Work out the finished part from the listing and answer in its coordinate system (mm). A direction names the side the tool comes from. Coordinates: 2 decimals unless noted, no trailing zeros. Order: outer loops, then holes, each group sorted by start corner. A loop starts at its lowest first (then second) coordinate and runs counter-clockwise, first axis right, second up.
1. Flat-ended cylindrical pins translate along their axes: pin 1 Ø1 at (x, y) = (26, -37) entering from -Z; pin 2 Ø6 at (x, z) = (-18.5, 24.5) entering from +Y; pin 3 Ø1.9 at (y, z) = (-31, 22) entering from -X; pin 4 Ø12 at (x, z) = (22.5, 22) entering from +Y. Find the tip coordinate at first contact, or state that the pin passes through.
2. The part is cut by section B-B, the plane z = 12.5. Give the vertices of the cut face in (x, y).
3. Find the intervals of material crossed by probe 1 along X at (y, z) = (-38, 7); probe 2 along X at (y, z) = (-35.75, 7.5); probe 3 along X at (y, z) = (-31, 19.5), in increasing order.
4. Determine the mould class of faces 4 (the flat face through (11, -30, 23)), 5 (the flat face through (0.6, -36.49, 12.92)), 6 (the cylindrical face through (-21.9, -32.5, 19.5)) for opening direction Z: +Z half, -Z half, draft (parallel to the pull), parting line (faces both ways), or undercut.
5. The part is cut by section A-A, the plane x = 3. Give the vertices of the cut face in (y, z), then the cut area to 3 significant figures.
6. A tool of negligible diameter and unlimited length cuts with its end or side. For faces 1 (the conical face through (-13.377, -33.758, 16.894)), 2 (the cylindrical face through (10.323, -32.344, 16.981)), 3 (the conical face through (-13.424, -29.345, 29.017)), from which of +Z, -Z, +X, -X, +Y, -Y can it reach the whole face along a straight path? Write none if from no direction.
```python
from build123d import *

# Parameters (mm, degrees)
SKETCH033_R             = 1.65
SKETCH033_R_2           = 3.7
PAD001_DEPTH            = 3
CHAMFER001_SIZE         = 2
CHAMFER002_SIZE         = 1.4
SKETCH035_R             = 1.5
POCKET009_DEPTH         = 1.5
BODY005_PLACEMENT_ANGLE = 340


with BuildPart() as part:
    # Sketch033 → Pad001 (new body)
    with BuildSketch(Plane.XZ):
        with BuildLine():
            Line((-33.808366, 37.4), (33.808366, 37.4))
            ThreePointArc((41.8, 29.765194), (39.33458, 35.18452), (33.808366, 37.4))
            Line((41.8, 29.765194), (42.65, 11.165194))
            ThreePointArc((34.658366, 2.8), (40.442878, 5.273779), (42.65, 11.165194))
            Line((34.658366, 2.8), (-34.658366, 2.8))
            ThreePointArc((-42.65, 11.165194), (-40.442878, 5.273779), (-34.658366, 2.8))
            Line((-42.65, 11.165194), (-41.8, 29.765194))
            ThreePointArc((-33.808366, 37.4), (-39.33458, 35.18452), (-41.8, 29.765194))
        make_face()
        with Locations((-36.75, 32.1)):
            Circle(SKETCH033_R, mode=Mode.SUBTRACT)
        with Locations((36.75, 32.1)):
            Circle(SKETCH033_R, mode=Mode.SUBTRACT)
        with Locations((-38, 8.1)):
            Circle(SKETCH033_R, mode=Mode.SUBTRACT)
        with Locations((38, 8.1)):
            Circle(SKETCH033_R, mode=Mode.SUBTRACT)
        with Locations((25.5, 23.3)):
            Circle(SKETCH033_R_2, mode=Mode.SUBTRACT)
        with BuildLine():
            Line((-11.25, 30.35), (8.75, 30.35))
            ThreePointArc((11, 28.1), (10.34099, 29.69099), (8.75, 30.35))
            Line((11, 28.1), (11, 19.5))
            ThreePointArc((8.75, 17.25), (10.34099, 17.90901), (11, 19.5))
            Line((8.75, 17.25), (-11.25, 17.25))
            ThreePointArc((-13.5, 19.5), (-12.84099, 17.90901), (-11.25, 17.25))
            Line((-13.5, 19.5), (-13.5, 28.1))
            ThreePointArc((-11.25, 30.35), (-12.84099, 29.69099), (-13.5, 28.1))
        make_face(mode=Mode.SUBTRACT)
        with BuildLine():
            Line((-30.35, 25.929165), (-25.65, 25.929165))
            ThreePointArc((-25.65, 14.670835), (-21.9, 20.3), (-25.65, 25.929165))
            Line((-30.35, 14.670835), (-25.65, 14.670835))
            ThreePointArc((-30.35, 25.929165), (-34.1, 20.3), (-30.35, 14.670835))
        make_face(mode=Mode.SUBTRACT)
    extrude(amount=PAD001_DEPTH)

    # Chamfer001
    chamfer001_edges = [part.edges().sort_by_distance(p)[0] for p in [
        (-1.25, -3, 30.35),
    ]]
    chamfer(chamfer001_edges, length=CHAMFER001_SIZE)

    # Chamfer002
    chamfer002_edges = [part.edges().sort_by_distance(p)[0] for p in [
        (-38.4, -3, 32.1),
        (-39.65, -3, 8.1),
        (35.1, -3, 32.1),
        (36.35, -3, 8.1),
    ]]
    chamfer(chamfer002_edges, length=CHAMFER002_SIZE)

    # Sketch035 → Pocket009 (cut)
    with BuildSketch(Plane.XZ):
        with Locations((25.5, 30.3)):
            Circle(SKETCH035_R)
    extrude(amount=POCKET009_DEPTH, mode=Mode.SUBTRACT)


with BuildPart() as part_1:
    # Body005 placement: moved
    add(part.part.moved(Location((0, -38, 0))).rotate(Axis((0, -38, 0), (1, 0, 0)), BODY005_PLACEMENT_ANGLE))


solid = part_1.part
```
Geometry says:
1. pin 1: stops at z = 2.63
1. pin 2: stops at y = -27.99
1. pin 3: stops at x = -42.15
1. pin 4: stops at y = -27.81
2. outline: (-42.6, -36.64) - (42.6, -36.64) - (42.55, -33.45) - (-42.55, -33.45) - close
3. probe 1: x = -41.45 to -39.91, -36.09 to 36.09, 39.91 to 41.45
3. probe 2: x = -42.08 to -39.63, -36.37 to 36.37, 39.63 to 42.08
3. probe 3: x = -42.21 to -34.09, -21.91 to -13.5, 11 to 22.85, 28.15 to 42.21
4. face 4: draft
4. face 5: +Z half
4. face 6: undercut
5. outline: (-39.86, 3.66) - (-37.04, 2.63) - (-32.1, 16.21) - (-33.04, 16.55) - (-35.6, 15.36) - close; (-29.75, 31.43) - (-28.56, 28.86) - (-27.62, 28.52) - (-25.21, 35.14) - (-28.03, 36.17) - close
5. area: 60.5 mm2
6. face 1: +Z, -Y
6. face 2: +Z, +Y
6. face 3: -Y
